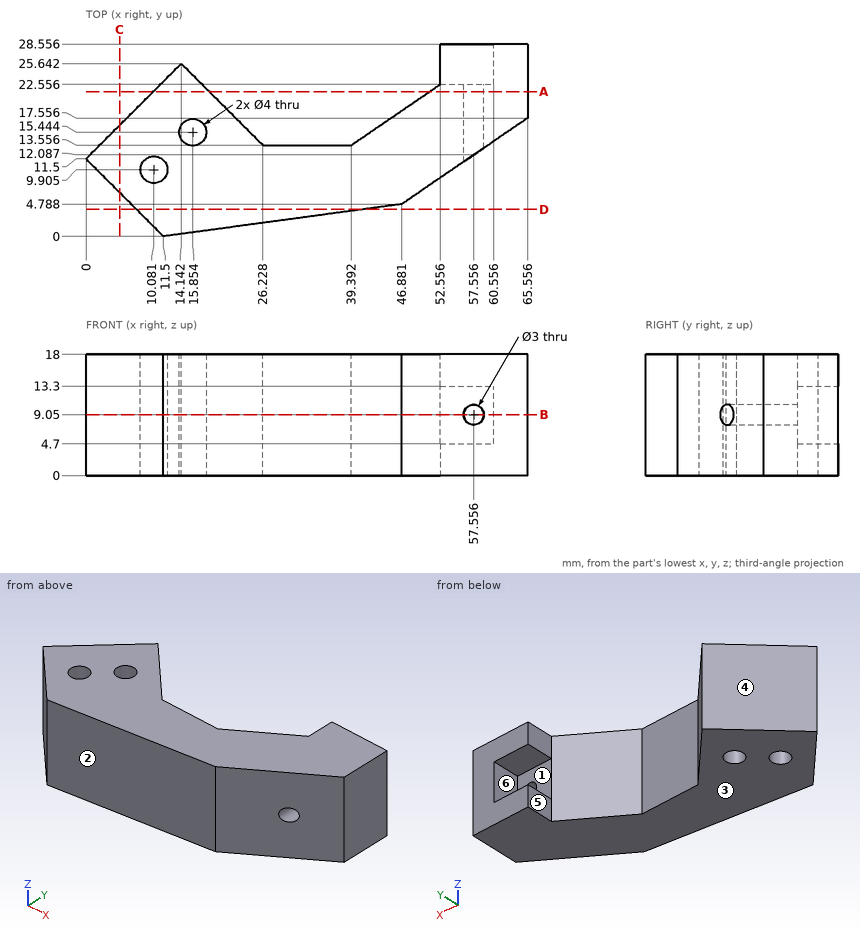
Print and shaded views of the part. All mm, measured from the part's lowest x, y and z. A direction names the side the tool comes from. Coordinates: 2 decimals unless noted, no trailing zeros. Order: outer loops, then holes, each group sorted by start corner. A loop starts at its lowest first (then second) coordinate and runs counter-clockwise, first axis right, second up. Notation, with made-up numbers: M -12,21.5 L 47,21.5 A31 cw 47,56.5 Z; hole C 20,59.5 d11. An arc over 180 degrees is marked long. Write each question's results on one line, items separated by ' | '. Start each with the question number.
Q1. Cut at A-A (y = 21.5). Count the separate pieces of the cut face and the enclosed holes in it, then the cut area to 3 significant figures.
Q2. Cut at D-D (y = 4). List the corners of the cut face in (x, z).
Q3. Pull direction Z, two halves, no side cores. Call the marked faces 1, 2 and 3: +Z half, -Z half, draft (parallel to the pull), parting line (faces both ways), or undercut.
Q4. Flat gauge pins, fed straight in: P1, Ø5, axis at x = 57.56, z = 9.05, coming from the +Y side; P2, Ø1.8, axis at y = 25, z = 10, coming from the -X side; P3, Ø1.4, axis at y = 27, z = 1.5, coming from the -X side. Where does each tip first touch, or does it go through?
Q5. Drill centre lines: probe 1 along Z at (x, y) = (60, 25.5); probe 2 along X at (y, z) = (21.5, 5.5) (1 decimal); probe 3 along Y at (x, z) = (14.5, 12) (1 decimal). Where is each one in solid material? Low to high. Write a range as from..to.
Q6. Which spindle directions (+Z, -Z, +X, -X, +Y, -Y) get a long thin tool onto all of the face, cutting with end or side? Do the marked faces 4, 5 and 6. Say none if no direction does.
Q7. Cut at C-C (x = 5). List the corners of the cut face in (y, z), then the cut area to 3 significant figures.
Q8. Cut at B-B (z = 9.05). List the corners of the cut face in (x, y) (1 decimal).
Found:
1) separate pieces: 2 | enclosed holes: 1 | area: 404 mm²
2) outline: M 7.5,0 L 41.06,0 L 41.06,18 L 7.5,18 Z
3) face 1: undercut | face 2: draft | face 3: -Z half
4) P1: y = 22.56 | P2: x = 12.6 | P3: x = 52.56
5) probe 1: 0..4.7, 13.3..18 | probe 2: 10..18.3, 51..65.6 | probe 3: 0.4..14, 16.9..25.3
6) face 4: +Z, -Z, -X, +Y | face 5: +Z, -Z, +Y | face 6: +Y
7) outline: M 6.5,0 L 16.5,0 L 16.5,18 L 6.5,18 Z | area: 180 mm²
8) outline: M 0,11.5 L 11.5,0 L 46.9,4.8 L 56.1,11.1 L 56.1,22.6 L 52.6,22.6 L 39.4,13.6 L 26.2,13.6 L 14.1,25.6 Z; M 59.1,13.1 L 65.6,17.6 L 65.6,28.6 L 60.6,28.6 L 60.6,22.6 L 59.1,22.6 Z; hole C 10.1,9.9 d4; hole C 15.9,15.4 d4
